from build123d import *

# Parameters (mm, degrees)
F1_DEPTH = 6.35
F3_DEPTH = 33.528
F4_R     = 7.812407
F5_DEPTH = 76.2


with BuildPart() as f1:
    # F0 (on Front) → F1 (new body)
    with BuildSketch(Plane.XZ):
        Polygon((0, 39.166801), (0, 0), (50.901599, 0), (32.613602, 39.166801), align=None)
    extrude(amount=-F1_DEPTH)

    # F2 (on face) → F3 (join)
    with BuildSketch(Plane.XZ):
        Polygon((45.216922, 0), (29.300908, 34.086801), (0, 34.086801), (0, 0), align=None)
    extrude(amount=F3_DEPTH)

    # F4 (on face) → F5 (cut)
    with BuildSketch(Plane(origin=(0, 0, 0), x_dir=(0, -1, 0), z_dir=(-1, 0, 0))):
        with Locations((16.764, 17.0434)):
            Circle(F4_R)
    extrude(amount=-F5_DEPTH, mode=Mode.SUBTRACT)


solid = f1.part
The listing builds one solid part. Answer for the finished solid, in the listing's coordinates (mm). A direction names the side the tool comes from. Give positions to 0.01 mm unless a question says otherwise; leave off trailing zeros. Loops run counter-clockwise (first coordinate to the right, second up) from the corner with the lowest first, then second, coordinate; pieces in that order, holes last. Notation, with made-up numbers: (-25, 29.25) - (4, 29.25) arc R21 ccw to (4, 49.25) - close; hole circle Ø7 at (0.25, -2). An arc over 180 degrees is marked (long way). Use one line per item in the form item = value.
1. Find the intervals of material crossed by line 1 along Y through (x, z) = (8, 17); line 2 along Z through (x, y) = (40, -17); line 3 along Z through (x, y) = (18, -16), in increasing order. Write a range as [from, to].
Calculated:
line_1 = [-33.53, -24.58], [-8.95, 6.35]
line_2 = [0, 9.23]
line_3 = [0, 9.27], [24.82, 34.09]
2. Section C-C on y = -19 is taken. Give the vertices of the cut face in (x, z).
Calculated:
outline = (0, 0) - (45.22, 0) - (40.75, 9.56) - (0, 9.56) - close; (0, 24.53) - (33.76, 24.53) - (29.3, 34.09) - (0, 34.09) - close
3. Given pin 1 Ø1 at (x, y) = (30, -16.5) entering from +Z; pin 2 Ø5 at (y, z) = (-7.5, 27.5) entering from +X, each flat-ended and moving along its own axis, determine where each tip first touches the part or whether it passes through.
Calculated:
pin_1 = 33.66
pin_2 = 33.54
4. Section D-D on x = 39 is taken. Give the vertices of the cut face in (y, z).
Calculated:
outline = (-33.53, 0) - (6.35, 0) - (6.35, 25.49) - (0, 25.49) - (0, 13.31) - (-9.9, 13.31) arc R7.81 cw to (-23.63, 13.31) - (-33.53, 13.31) - close
5. Section A-A on z = 21.5 is taken. Give the vertices of the cut face in (x, y), then the cut area to 3 significant figures.
Calculated:
outline = (0, -33.53) - (35.18, -33.53) - (35.18, -23.18) - (0, -23.18) - close; (0, -10.35) - (35.18, -10.35) - (35.18, 0) - (40.86, 0) - (40.86, 6.35) - (0, 6.35) - close
area = 987 mm^2
6. Which of the six approach directions +Z, -Z, +X, -X, +Y, -Y give full straight-line access (tool end or side, diameter ignored) to faces 5 (the face through (39.139, -9.079, 13.017)), 6 (the face through (15, -17, 34.087)), 7 (the face through (41.886, 3.131, 19.309))?
Calculated:
face_5 = +Z, +X, -Y
face_6 = +Z, +X, -X, -Y
face_7 = +Z, +X, +Y, -Y
7. Section B-B on x = 9 is taken. Give the vertices of the cut face in (y, z), then the cut area to 3 significant figures.
Calculated:
outline = (-33.53, 0) - (6.35, 0) - (6.35, 39.17) - (0, 39.17) - (0, 34.09) - (-33.53, 34.09) - close; hole circle Ø15.62 at (-16.76, 17.04)
area = 1,200 mm^2
8. The mould has two halves that part along Y. Classify faces 1 (the face through (19, 6.35, 20)), 2 (the face through (20.21, -15.07, 9.417)), 3 (the face through (17, -33.528, 17)), 4 (the face through (0, -9, 20)): pulls with the +Y half, pulls with the -Y half, needs draft (parallel to the pull), parting line crosses it, or undercut.
Calculated:
face_1 = pulls with the +Y half
face_2 = undercut
face_3 = pulls with the -Y half
face_4 = needs draft
